Work out the finished part from the listing and answer in its coordinate system (mm). Face numbers are marked on the shaded views. Give positions to 0.01 mm unless a question says otherwise; leave off trailing zeros. Write each loop counter-clockwise with the first axis right and the second up, starting at its lowest first coordinate (ties: lowest second). Pieces come first, ordered by that corner, then holes.
1) Straight lines are drawn through the part: probe 1 along X at (y, z) = (30, 48); probe 2 along Y at (x, z) = (20, 6); probe 3 along X at (y, z) = (27, 50). For each, find the intervals that lie inside material, in ascending order.
2) Determine the mould class of the marked faces 1, 2 and 3 for opening direction Y: pulls with the +Y half, pulls with the -Y half, needs draft (parallel to the pull), parting line crosses it, or undercut.
3) Find section B-B (y = 37.5). Determine the outline of the cut face in (x, z), plus the area to 3 significant figures.
4) Find section A-A (x = 25). Determine the outline of the cut face in (y, z).
```python
from build123d import *

# Parameters (mm, degrees)
F0_W        = 51.974568516
F0_H        = 66.7630434036
F0_R        = 13.7134635275
F1_DEPTH    = 59.80942
F2_SIZE     = 5.08
F3_T1_DEPTH = 123.30942


# Not quite as in the source:
# - a fillet or chamfer that OpenCascade refuses, or shapes differently, is made with other operations: its cross-section is extruded or revolved along the edge and cut away or added


with BuildPart() as f1:
    # F0 (on Top) → F1 (new body)
    with BuildSketch(Plane.XY):
        with Locations((25.987284258, 33.3815217018)):
            Rectangle(F0_W, F0_H)
        with Locations((24.4355015457, 35.2227129042)):
            Circle(F0_R, mode=Mode.SUBTRACT)
    extrude(amount=F1_DEPTH)

    # F2
    f2_edges = [f1.edges().sort_by_distance(p)[0] for p in [
        (51.974569, 0, 29.90471),
    ]]
    chamfer(f2_edges, length=F2_SIZE)

    # F3: fillet of radius 12.7 on 1 edges, made by hand

    # F3_s2 → F3_t1 (cut)
    with BuildSketch(Plane.XY.offset(-31.75)):
        with BuildLine():
            add(Edge.make_bspline(
                [(51.974568516, 54.0630434036), (51.974568516, 66.7630434036), (39.274568516, 66.7630434036)],
                knots=[0, 0, 0, 1, 1, 1], degree=2, weights=[1, 4, 1]))
            Line((39.274568516, 66.7630434036), (51.974568516, 66.7630434036))
            Line((51.974568516, 66.7630434036), (51.974568516, 54.0630434036))
        make_face()
    extrude(amount=F3_T1_DEPTH, mode=Mode.SUBTRACT)


solid = f1.part
```
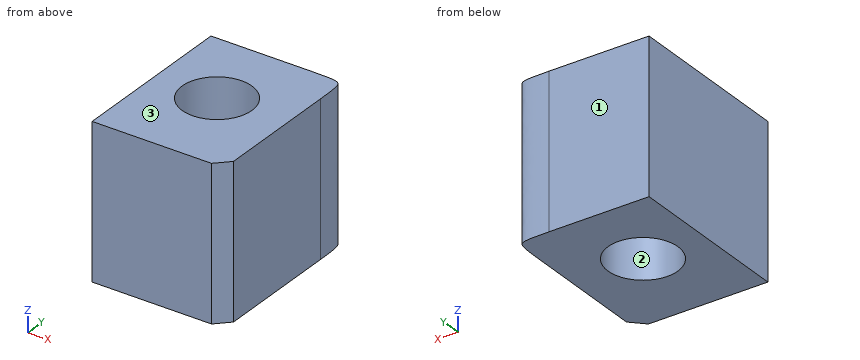
Results:
1. probe 1: x = 0 to 11.76, 37.12 to 51.97
1. probe 2: y = 0 to 22.25, 48.2 to 66.76
1. probe 3: x = 0 to 13.46, 35.41 to 51.97
2. face 1: pulls with the +Y half
2. face 2: undercut
2. face 3: needs draft
3. outline: (0, 0) - (10.91, 0) - (10.91, 59.81) - (0, 59.81) - close; (37.96, 0) - (51.97, 0) - (51.97, 59.81) - (37.96, 59.81) - close
3. area: 1,490 mm2
4. outline: (0, 0) - (21.52, 0) - (21.52, 59.81) - (0, 59.81) - close; (48.92, 0) - (66.76, 0) - (66.76, 59.81) - (48.92, 59.81) - close
